Here's the drawing with two shaded views (mm, measured from the low corner). I have some questions. Round coordinates to 2 decimals unless told otherwise and drop trailing zeros. Write each loop counter-clockwise with the first axis right and the second up, starting at its lowest first coordinate (ties: lowest second). Pieces come first, ordered by that corner, then holes. Notation, with made-up numbers: M 3.5,79 L 53.5,79 A26 ccw 53.5,102 Z; hole C 57,-8 d4. An arc over 180 degrees is marked long. Write item = value, one per line. Start each with the question number.
(1) I want a section at A-A (x = 31.75). List the corners of the cut face in (y, z) for me.
(2) I want a section at D-D (x = 95.25). List the corners of the cut face in (y, z) for me (1 decimal).
(3) I need wall thicknesses on line 1 along X through (y, z) = (7.62, 56.75) (1 decimal); line 2 along X through (y, z) = (11.5, 35) (1 decimal); line 3 along Z through (x, y) = (92.5, 6.25). Which ranges of each line are inside material? Lowest first, please.
(4) I want a section at B-B (z = 31.75). List the corners of the cut face in (x, y) for me (1 decimal), and give its area (3 significant figures).
(5) I want a section at C-C (y = 11). Give the number of separate pieces and of enclosed holes in the cut face, and give its area (3 significant figures).
(6) Will these pins go through, and if not, where does the flat tip stop? pin 1 Ø2.5 at (x, y) = (13.843, 7.62) entering from +Z (1 decimal); pin 2 Ø2.5 at (x, z) = (38.89, 19.38) entering from -Y; pin 3 Ø3.5 at (x, y) = (62.103, 7.62) entering from +Z (1 decimal).
(7) If we mould it in two halves opening along X, with no side actions, what happens to the marked faces 1, 2, 3 and 4? For each: released by +X, released by -X, zero draft, split by the parting line, or undercut.
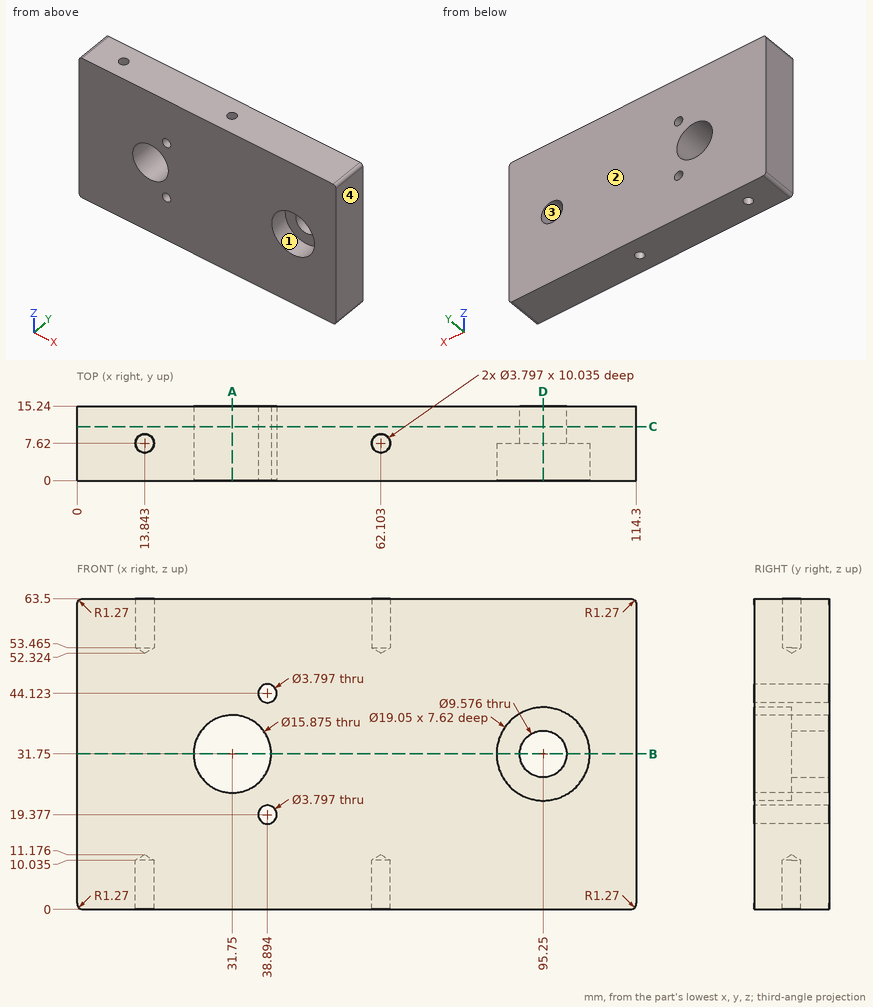
Returned:
q1.outline = M 0,0 L 15.24,0 L 15.24,23.81 L 0,23.81 Z; M 0,39.69 L 15.24,39.69 L 15.24,63.5 L 0,63.5 Z
q2.outline = M 0,0 L 15.2,0 L 15.2,27 L 7.6,27 L 7.6,22.2 L 0,22.2 Z; M 0,41.3 L 7.6,41.3 L 7.6,36.5 L 15.2,36.5 L 15.2,63.5 L 0,63.5 Z
q3.line_1 = 0 to 11.9, 15.7 to 60.2, 64 to 114.3
q3.line_2 = 0 to 24.5, 39 to 91.7, 98.8 to 114.3
q3.line_3 = 0 to 22.63, 40.87 to 63.5
q4.outline = M 0,0 L 23.8,0 L 23.8,15.2 L 0,15.2 Z; M 39.7,0 L 85.7,0 L 85.7,7.6 L 90.5,7.6 L 90.5,15.2 L 39.7,15.2 Z; M 100,7.6 L 104.8,7.6 L 104.8,0 L 114.3,0 L 114.3,15.2 L 100,15.2 Z
q4.area = 1,280 mm²
q5.separate_pieces = 1
q5.enclosed_holes = 4
q5.area = 6,960 mm²
q6.pin_1 = 53.1
q6.pin_2 = through
q6.pin_3 = 53.4
q7.face_1 = undercut
q7.face_2 = zero draft
q7.face_3 = undercut
q7.face_4 = released by +X
